```python
from build123d import *

# Parameters (mm, degrees)
BOSS_EXTRUDE1_DEPTH = 50
BOSS_EXTRUDE2_DEPTH = 3
CIRPATTERN1_COUNT   = 2
CHAMFER1_SIZE       = 1
FILLET1_R           = 0.5
CHAMFER2_START      = -1
CHAMFER2_DEPTH      = 10


with BuildPart() as part:
    # Sketch2 → Boss-Extrude1 (new body)
    with BuildSketch(Plane.XY):
        Polygon((0, 0), (0, 7.65), (14, 7.65), (14, 5.65), (2, 5.65), (2, 2), (14, 2), (14, 0), align=None)
    extrude(amount=BOSS_EXTRUDE1_DEPTH)

    # Sketch3 → Boss-Extrude2 (add)
    with BuildSketch(Plane(origin=(0, 7.65, 0), x_dir=(1, 0, 0), z_dir=(0, 1, 0))):
        with BuildLine():
            Line((0, -2.7), (0, -1.5))
            Line((0, -1.5), (-3.920792386, -1.5))
            Line((-3.920792386, -1.5), (-4.935568127, -5.287194625))
            Line((-4.935568127, -5.287194625), (-5.804901371, -5.054257484))
            Line((-5.804901371, -5.054257484), (-8.202748881, -14.003146224))
            Line((-8.202748881, -14.003146224), (-7.333415638, -14.236083364))
            Line((-7.333415638, -14.236083364), (-8.886329908, -20.031638322))
            Line((-8.886329908, -20.031638322), (-9.755663152, -19.798701181))
            Line((-9.755663152, -19.798701181), (-15.776457135, -42.268610229))
            ThreePointArc((-15.776457135, -42.268610229), (-15.776457135, -48.064165187), (-12.878679656, -43.045067364))
            Line((-12.878679656, -43.045067364), (-6.857885673, -20.575158317))
            Line((-6.857885673, -20.575158317), (-7.727218917, -20.342221176))
            Line((-7.727218917, -20.342221176), (-6.174304646, -14.546666218))
            Line((-6.174304646, -14.546666218), (-5.304971403, -14.779603359))
            Line((-5.304971403, -14.779603359), (-4.916742835, -13.330714619))
            Line((-4.916742835, -13.330714619), (-0.75, -13.330714619))
            Line((-0.75, -13.330714619), (-0.75, -10.330714619))
            Line((-0.75, -10.330714619), (-4.112895258, -10.330714619))
            Line((-4.112895258, -10.330714619), (-2.907123892, -5.830714619))
            Line((-2.907123892, -5.830714619), (-3.776457135, -5.597777479))
            Line((-3.776457135, -5.597777479), (-3, -2.7))
            Line((-3, -2.7), (0, -2.7))
        make_face()
    boss_extrude2 = extrude(amount=-BOSS_EXTRUDE2_DEPTH)

    # CirPattern1: Boss-Extrude2 ×2 about axis
    cirpattern1_axis = Axis((0, 3.825, 25), (1, 0, 0))
    for i in range(1, CIRPATTERN1_COUNT):
        add(boss_extrude2.rotate(cirpattern1_axis, i * 360 / CIRPATTERN1_COUNT))

    # Chamfer1
    chamfer1_edges = [part.edges().sort_by_distance(p)[0] for p in [
        (0, 7.65, 26.35),
        (14, 7.65, 25),
        (0, 7.65, 0.75),
        (7, 7.65, 50),
        (7, 7.65, 0),
    ]]
    chamfer(chamfer1_edges, length=CHAMFER1_SIZE)

    # Fillet1
    fillet1_edges = [part.edges().sort_by_distance(p)[0] for p in [
        (-8.886329908, 6.15, 20.031638322),
        (-7.333415638, 6.15, 14.236083364),
        (-4.935568127, 6.15, 5.287194625),
        (-3.920792386, 6.15, 1.5),
        (0, 5.65, 1.5),
        (0, 5.65, 2.7),
        (-3, 6.15, 2.7),
        (-3.776457135, 6.15, 5.597777479),
        (-6.174304646, 6.15, 14.546666218),
        (-7.727218917, 6.15, 20.342221176),
        (-8.886329908, 1.5, 29.968361678),
        (-7.333415638, 1.5, 35.763916636),
        (-4.935568127, 1.5, 44.712805375),
        (-3.920792386, 1.5, 48.5),
        (0, 1.5, 48.5),
        (0, 1.5, 47.3),
        (-3, 1.5, 47.3),
        (-3.776457135, 1.5, 44.402222521),
        (-6.174304646, 1.5, 35.453333782),
        (-7.727218917, 1.5, 29.657778824),
    ]]
    fillet(fillet1_edges, radius=FILLET1_R)

    # Chamfer2: read off the stored shape, not the designer's step
    # Chamfer2 outline → Chamfer2 (cut)
    with BuildSketch(Plane(origin=(0, 0, 0), x_dir=(1, 0, 0), z_dir=(0, 1, 0)).offset(CHAMFER2_START)):
        with BuildLine():
            Line((-7.464876997, -38.750629138), (-7.733281129, -35.862956659))
            ThreePointArc((-7.733281129, -35.862956659), (-7.7741568, -35.879982991), (-7.816378551, -35.893326158))
            Line((-7.816378551, -35.893326158), (-8.202748881, -35.996853776))
            Line((-8.202748881, -35.996853776), (-7.464876997, -38.750629138))
        make_face()
        with BuildLine():
            Line((-7.733281129, -14.137043341), (-7.464876997, -11.249370862))
            Line((-7.464876997, -11.249370862), (-8.202748881, -14.003146224))
            Line((-8.202748881, -14.003146224), (-7.816378551, -14.106673842))
            ThreePointArc((-7.816378551, -14.106673842), (-7.7741568, -14.120017009), (-7.733281129, -14.137043341))
        make_face()
    extrude(amount=CHAMFER2_DEPTH, mode=Mode.SUBTRACT)


solid = part.part
```
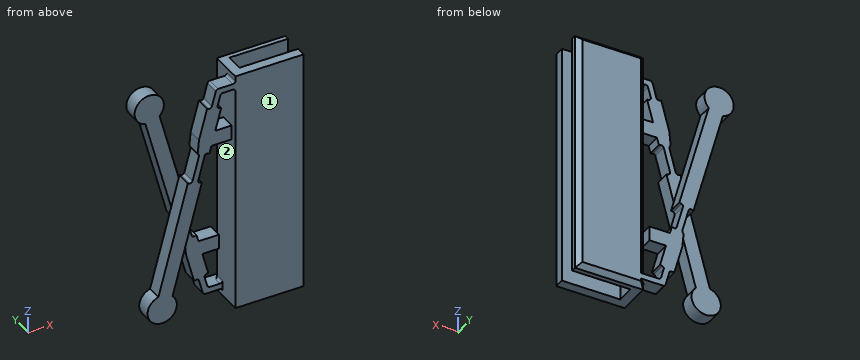
Work out the finished part from the listing and answer in its coordinate system (mm). Face numbers are marked on the shaded views. Give positions to 0.01 mm unless a question says otherwise; leave off trailing zeros. Loops run counter-clockwise (first coordinate to the right, second up) from the corner with the lowest first, then second, coordinate; pieces in that order, holes last. Notation, with made-up numbers: (45.25, 13.25) -> (60.25, 13.25) arc R21 ccw to (60.25, 38.25) -> close; hole circle Ø8 at (-22, -40). An arc over 180 degrees is marked (long way). Write item = value, one per line. Start each with the question number.
(1) The mould has two halves that part along X. Classify the marked faces 1 and 2: +X half, -X half, draft (parallel to the pull), parting line (faces both ways), or undercut.
(2) Find section C-C on x = -15. Give the vertices of the cut face in (y, z).
(3) Find the intervals of material crossed by probe 1 along Y at (x, z) = (5, 44); probe 2 along X at (y, z) = (7.25, 4); probe 3 along X at (y, z) = (6.5, 32.5), in increasing order. Write a range as from..to.
(4) Given pin 1 Ø2 at (y, z) = (2, 23) entering from -X; pin 2 Ø0.9 at (x, y) = (-2, 1.5) entering from +Z; pin 3 Ø1.8 at (y, z) = (4, 26.5) entering from +X, each flat-ended and moving along its own axis, determine where each tip first touches the part or whether it passes through.
(5) Find section A-A on x = 10. Give the vertices of the cut face in (y, z).
(6) Find section B-B on z = 34. Give the vertices of the cut face in (x, y).
From the geometry:
q1.face_1 = draft
q1.face_2 = undercut
q2.outline = (0, 1.83) -> (3, 1.83) -> (3, 10.63) -> (0, 10.63) -> close; (4.65, 39.37) -> (7.65, 39.37) -> (7.65, 48.17) -> (4.65, 48.17) -> close
q3.probe_1 = 0..2, 5.65..7.65
q3.probe_2 = -4.59..-3.35, 0.6..13.4
q3.probe_3 = -13.16..-10.05, 0..14
q4.pin_1 = -11.95
q4.pin_2 = 48.5
q4.pin_3 = 2
q5.outline = (0, 0) -> (2, 0) -> (2, 50) -> (0, 50) -> close; (5.65, 0) -> (6.65, 0) -> (7.65, 1) -> (7.65, 49) -> (6.65, 50) -> (5.65, 50) -> close
q6.outline = (-13.56, 4.65) -> (-10.46, 4.65) -> (-10.46, 7.65) -> (-13.56, 7.65) -> close; (-7.81, 0) -> (-6.56, 0) -> (-6.56, 3) -> (-7.81, 3) -> close; (0, 0) -> (14, 0) -> (14, 2) -> (2, 2) -> (2, 5.65) -> (14, 5.65) -> (14, 6.65) -> (13, 7.65) -> (1, 7.65) -> (0, 6.65) -> close
